Autodesk Inventor part; units mm, degrees
ref_plane "YZ Plane" through (0, 0, 0) normal (1, 0, 0) x (0, 1, 0)
ref_plane "XZ Plane" through (0, 0, 0) normal (0, 1, 0) x (-1, 0, 0)
ref_plane "XY Plane" through (0, 0, 0) normal (0, 0, 1) x (1, 0, 0)
sketch "Sketch1" plane through (0, 0, 0) normal (0, 1, 0) x (-1, 0, 0)
  line L0 (15, 17.8107) -> (15, 41.4147) construction
  line L1 (30, 60.5) -> (30, 0)
  line L2 (25, 17.5) -> (25, 26)
  line L3 (25, 26) -> (24, 26)
  line L4 (24, 26) -> (24, 17.5)
  line L5 (24, 17.5) -> (25, 17.5)
  line L6 (24, 34.5) -> (25, 34.5)
  line L7 (25, 34.5) -> (25, 43)
  line L8 (25, 43) -> (24, 43)
  line L9 (24, 43) -> (24, 34.5)
  line L10 (25, 57.75) -> (25, 60.5)
  line L11 (25, 60.5) -> (30, 60.5)
  line L12 (10, 57.75) -> (10, 60.5)
  line L13 (25, 57.75) -> (10, 57.75)
  line L14 (25, 2.75) -> (25, 0)
  line L15 (25, 0) -> (30, 0)
  line L16 (10, 2.75) -> (10, 0)
  line L17 (25, 2.75) -> (10, 2.75)
  line L18 (0, 50.75) -> (-2.75, 50.75)
  line L19 (-2.75, 50.75) -> (-2.75, 43.75)
  line L20 (-2.75, 43.75) -> (0, 43.75)
  line L21 (0, 16.75) -> (-2.75, 16.75)
  line L22 (-2.75, 16.75) -> (-2.75, 9.75)
  line L23 (-2.75, 9.75) -> (0, 9.75)
  line L24 (17.3275, 30.25) -> (11.5049, 30.25) construction
  line L25 (0, 50.75) -> (0, 57.75)
  line L26 (0, 2.75) -> (0, 9.75)
  line L27 (0, 16.75) -> (0, 43.75)
  line L28 (10, 0) -> (5, 0)
  line L29 (5, 0) -> (5, 2.75)
  line L30 (5, 2.75) -> (0, 2.75)
  line L31 (10, 60.5) -> (5, 60.5)
  line L32 (5, 60.5) -> (5, 57.75)
  line L33 (5, 57.75) -> (0, 57.75)
  point P0 (0, 0)
  point P1 (0, 0)
  point P2 (0, 0)
  point P3 (0, 0)
  point P4 (0, 0)
  point P5 (25.5, 47.25)
  point P6 (25.5, 30.25)
  point P7 (25.5, 13.25)
  dimension "d151" = 8.5
  dimension "d153" = 1
  dimension "d155" = 5
  dimension "d159" = 17
  dimension "d160" = 17
  dimension "d161" = 4.25
  dimension "d162" = 4.25
  dimension "d176" = 4.5
  dimension "d177" = 5
  dimension "d179" = 55
  dimension "d180" = 2.75
  dimension "d182" = 7
  dimension "d183" = 7
  dimension "d184" = 30
extrude "Extrusion1" add sketch "Sketch1" against normal blind 1.5
hole "Hole1" at (-25.5, 0, 47.25) at (-25.5, 0, 30.25) at (-25.5, 0, 13.25) direction (0, -1, 0) diameter 1 end through all
sketch "Sketch4" plane through (0, 0, 0) normal (0, 1, 0) x (1, 0, 0)
  line L0 (-3, -46.55) -> (-3, -3.25)
  line L1 (-3, -3.25) -> (-21, -3.25)
  line L2 (-21, -3.25) -> (-21, -46.55)
  line L3 (-21, -46.55) -> (-3, -46.55)
  line L4 (-25, -2.75) -> (-10, -2.75)
  line L5 (-10, -2.75) -> (-25, -2.75)
  line L6 (0, -43.75) -> (0, -16.75)
  point P0 (0, 0)
  dimension "d188" = 43.3
  dimension "d189" = 18
  dimension "d190" = 3
  dimension "d212" = 0.5
extrude "Extrusion11" add sketch "Sketch4" along normal blind 5
sketch "Sketch6" plane through (0, 5, 0) normal (0, 1, 0) x (1, 0, 0)
  line L0 (-17.0504, -18.7342) -> (-12.1007, -13.7844)
  line L1 (-12.1007, -13.7844) -> (-7.1509, -18.7342)
  line L2 (-7.1509, -18.7342) -> (-12.1007, -23.6839)
  line L3 (-12.1007, -23.6839) -> (-17.0504, -18.7342)
  point P0 (0, 0)
  dimension "d198" = 7
  dimension "d199" = 7
extrude "Extrusion13" add sketch "Sketch6" along normal blind 2
sketch "Sketch7" plane through (0, 5, 0) normal (0, 1, 0) x (1, 0, 0)
  line L0 (-15.6959, -40.3292) -> (-8.6959, -40.3292)
  line L1 (-8.6959, -40.3292) -> (-8.6959, -45.3292)
  line L2 (-8.6959, -45.3292) -> (-15.6959, -45.3292)
  line L3 (-15.6959, -45.3292) -> (-15.6959, -40.3292)
  point P0 (0, 0)
  dimension "d202" = 7
  dimension "d203" = 5
extrude "Extrusion14" add sketch "Sketch7" along normal blind 2.5
sketch "Sketch8" plane through (0, 7.5, 0) normal (0, 1, 0) x (1, 0, 0)
  line L0 (-15.3142, -41.2282) -> (-14.6142, -41.2282)
  line L1 (-14.6142, -41.2282) -> (-14.6142, -41.9282)
  line L2 (-14.6142, -41.9282) -> (-15.3142, -41.9282)
  line L3 (-15.3142, -41.9282) -> (-15.3142, -41.2282)
  line L4 (-15.3142, -43.9282) -> (-14.6142, -43.9282)
  line L5 (-14.6142, -43.9282) -> (-14.6142, -44.6282)
  line L6 (-14.6142, -44.6282) -> (-15.3142, -44.6282)
  line L7 (-15.3142, -44.6282) -> (-15.3142, -43.9282)
  line L8 (-12.6142, -41.2282) -> (-11.9142, -41.2282)
  line L9 (-11.9142, -41.2282) -> (-11.9142, -41.9282)
  line L10 (-11.9142, -41.9282) -> (-12.6142, -41.9282)
  line L11 (-12.6142, -41.9282) -> (-12.6142, -41.2282)
  line L12 (-12.6142, -43.9282) -> (-11.9142, -43.9282)
  line L13 (-11.9142, -43.9282) -> (-11.9142, -44.6282)
  line L14 (-11.9142, -44.6282) -> (-12.6142, -44.6282)
  line L15 (-12.6142, -44.6282) -> (-12.6142, -43.9282)
  line L16 (-9.9142, -41.2282) -> (-9.2142, -41.2282)
  line L17 (-9.2142, -41.2282) -> (-9.2142, -41.9282)
  line L18 (-9.2142, -41.9282) -> (-9.9142, -41.9282)
  line L19 (-9.9142, -41.9282) -> (-9.9142, -41.2282)
  line L20 (-9.9142, -43.9282) -> (-9.2142, -43.9282)
  line L21 (-9.2142, -43.9282) -> (-9.2142, -44.6282)
  line L22 (-9.2142, -44.6282) -> (-9.9142, -44.6282)
  line L23 (-9.9142, -44.6282) -> (-9.9142, -43.9282)
  point P0 (0, 0)
  dimension "d206" = 0.7
  dimension "d207" = 2
  dimension "d208" = 2
  dimension "d209" = 2
extrude "Extrusion15" add sketch "Sketch8" along normal blind 5
sketch "Sketch9" plane through (-3, 0, 3.25) normal (0, 0, -1) x (-1, 0, 0)
  line L0 (12.75, 8.5) -> (5.25, 8.5)
  line L1 (5.25, 8.5) -> (5.25, 5)
  line L2 (5.25, 5) -> (12.75, 5)
  line L3 (12.75, 5) -> (12.75, 8.5)
  line L4 (9, 5.7242) -> (9, 7.4058) construction
  line L5 (18, 0) -> (18, 5)
  line L6 (0, 5) -> (18, 5)
  point P0 (-3, 0)
  dimension "d213" = 7.5
  dimension "d214" = 3.5
  dimension "d215" = 9
extrude "Extrusion16" add sketch "Sketch9" along normal blind 2 and the other way blind 7
sketch "Sketch15" plane through (-3, 0, 1.25) normal (0, 0, -1) x (-1, 0, 0)
  line L0 (12.25, 8.25) -> (5.75, 8.25)
  line L1 (5.75, 8.25) -> (5.75, 5.25)
  line L2 (5.75, 5.25) -> (12.25, 5.25)
  line L3 (12.25, 5.25) -> (12.25, 8.25)
  line L4 (5.25, 8.5) -> (5.25, 5)
  line L5 (12.75, 8.5) -> (5.25, 8.5)
  point P0 (-3, 0)
  dimension "d242" = 6.5
  dimension "d243" = 3
  dimension "d244" = 0.5
  dimension "d245" = 0.25
extrude "Extrusion20" cut sketch "Sketch15" against normal blind 5
properties part number "Motherboard_dummy" material "ABS Plastic"
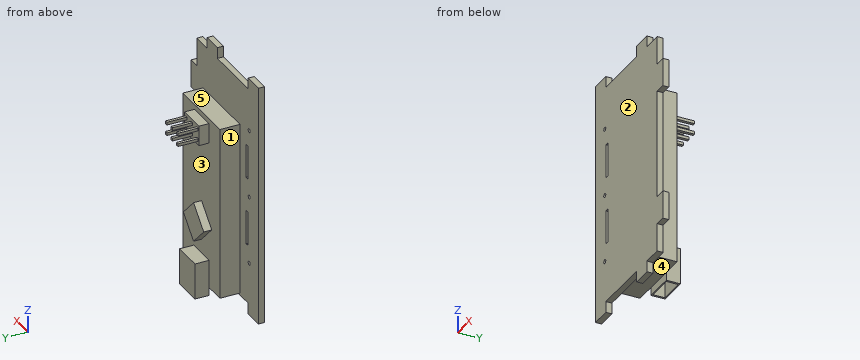
Verification items for the finished model (mm, model axes). Face numbers are marked on the shaded views. A direction names the side the tool comes from. Coordinates: 2 decimals unless noted, no trailing zeros. Order: outer loops, then holes, each group sorted by start corner. A loop starts at its lowest first (then second) coordinate and runs counter-clockwise, first axis right, second up. Notation, with made-up numbers: M 72,36 L 128,36 A33 ccw 128,72 Z; hole C 58,53 d8. An arc over 180 degrees is marked long. Return JSON: item names as keys, results as strings.
1) Cross-section at D-D, the plane y = 1.5. Record the boundary of the cut face in (x, z), and give its area (3 significant figures).
Answer list:
{"outline": "M -21,3.25 L -3,3.25 L -3,46.55 L -21,46.55 Z", "area": "779 mm2"}
2) Thickness scan on L1, parallel to X at y = 10.5, z = 41.5; L2, parallel to Z at x = -25.5, y = -1; L3, parallel to X at y = -0.5, z = 47.25. Record the ranges inside material, lowest first. Write a range as [from, to].
Answer list:
{"L1": "[-15.31, -14.61], [-12.61, -11.91], [-9.91, -9.21]", "L2": "[0, 12.75], [13.75, 29.75], [30.75, 46.75], [47.75, 60.5]", "L3": "[-30, -26], [-25, 2.75]"}
3) Cross-section at C-C, the plane z = 53. Record the boundary of the cut face in (x, y).
Answer list:
{"outline": "M -30,-1.5 L 0,-1.5 L 0,0 L -30,0 Z"}
4) Access from +Z, -Z, +X, -X, +Y, -Y to the whole of each face (thin tool, end or side, straight path). Record for the marked faces 1 and 2.
Answer list:
{"face 1": "+Z, -Z, -X, +Y", "face 2": "+Z, -Z, +X, -X, -Y"}
5) Release check for a two-part mould opening along Z. For the marked faces 3, 4 and 5 record: +Z half, -Z half, draft (parallel to the pull), parting line (faces both ways), or undercut.
Answer list:
{"face 3": "undercut", "face 4": "-Z half", "face 5": "+Z half"}
6) Gauge pin test, flat ends, axial feed: pin 1 (6 mm diameter, centred on x = -26.5, z = 27.5, fed in from +Y); pin 2 (5 mm diameter, centred on x = -9.5, z = 15.5, fed in from +Y); pin 3 (3 mm diameter, centred on x = -21.5, y = 5.5, fed in from +Z); pin 4 (8 mm diameter, centred on y = 10, z = 33, fed in from -X). Record the tip position at first contact, or that the pin passes through.
Answer list:
{"pin 1": "y = 0", "pin 2": "y = 7", "pin 3": "z = 46.55", "pin 4": "through"}
7) Cross-section at B-B, the plane x = -19. Record the boundary of the cut face in (y, z), and give its area (3 significant figures).
Answer list:
{"outline": "M -1.5,2.75 L 0,2.75 L 0,3.25 L 5,3.25 L 5,46.55 L 0,46.55 L 0,57.75 L -1.5,57.75 Z", "area": "299 mm2"}
8) Cross-section at A-A, the plane y = 10.25. Record the boundary of the cut face in (x, z), and give its area (3 significant figures).
Answer list:
{"outline": "M -15.31,41.23 L -14.61,41.23 L -14.61,41.93 L -15.31,41.93 Z; M -15.31,43.93 L -14.61,43.93 L -14.61,44.63 L -15.31,44.63 Z; M -12.61,41.23 L -11.91,41.23 L -11.91,41.93 L -12.61,41.93 Z; M -12.61,43.93 L -11.91,43.93 L -11.91,44.63 L -12.61,44.63 Z; M -9.91,41.23 L -9.21,41.23 L -9.21,41.93 L -9.91,41.93 Z; M -9.91,43.93 L -9.21,43.93 L -9.21,44.63 L -9.91,44.63 Z", "area": "2.94 mm2"}
